Can you work these out from the model? Positions are in its coordinate system, mm. A direction names the side the tool comes from. Coordinates: 2 decimals unless noted, no trailing zeros. Loops run counter-clockwise (first coordinate to the right, second up) from the corner with the lowest first, then second, coordinate; pieces in that order, holes last. Notation, with made-up numbers: M -15.5,-13 L 41.5,-13 A19 ccw 41.5,11 Z; hole C 68,-9 d5. An arc over 180 degrees is marked long. Answer as a JSON object with one key per item and string values. Group by question number.
Item 1: We'd pull the mould along Y, two halves only. Please class faces 1 (the flat face through (0, -2, -22)), 2 (the cylindrical face through (-1.57, -3.86, 5.04)), 3 (the flat face through (-1.565, -54.056, 3.924)): +Y half, -Y half, draft (parallel to the pull), parting line (faces both ways), or undercut.
Item 2: Which directions (+Z, -Z, +X, -X, +Y, -Y) give clear straight access to the entire face, cutting with the end or side of a thin tool? Please do faces 4 (the cylindrical face through (-1.565, -46.994, -15.824)), 5 (the flat face through (-1.565, -44.442, -47.356)).
Item 3: I'm going to push flat-ended pins straight in: pin 1 Ø1 at (x, y) = (-2.5, -20.5) entering from +Z; pin 2 Ø1.5 at (y, z) = (75.5, -40) entering from -X. Where does each tip first touch, or does it pass through?
Item 4: Suppose I cut it at C-C (z = -56.5). Write out the boundary of the cut face in (x, y) (3 decimals).
Item 5: Suppose I cut it at D-D (x = -2.5). Write out the boundary of the cut face in (y, z).
Item 6: If I drill on line 1 (Y direction, x = -0.7, z = -25); line 2 (Y direction, x = -2.7, z = 2.5); line 3 (Y direction, x = -2.15, z = 2), over which ranges is the centre line in solid material (lowest first)?
Item 7: Suppose I cut it at B-B (z = -44). Write out the boundary of the cut face in (x, y) (3 decimals).
Item 8: Suppose I cut it at A-A (y = 0). Write out the boundary of the cut face in (x, z) (3 decimals), then the cut area to 3 significant figures.
```python
from build123d import *

# Parameters (mm, degrees)
SKETCH1_R           = 6.35
SKETCH1_R_2         = 5
BOSS_EXTRUDE1_DEPTH = 3.175


with BuildPart() as part:
    # Sketch1 → Boss-Extrude1 (new body)
    with BuildSketch(Plane.YZ):
        Polygon((-92.963597619, -40.991822572), (-82.715641976, -64.232721977), (-5.080718921, -30), (2.443726878, -30), (78.037119616, -69.842164643), (89.880151319, -47.372126813), (101.723183023, -24.902088983), (7.042880264, 25), (-6.258566793, 25), (-103.211553262, -17.750923167), align=None)
        with Locations(Location((0, 0, 0), (0, 0, 270))):
            Circle(SKETCH1_R, mode=Mode.SUBTRACT)
        with Locations(Location((-81.343147916, -35.867844751, 0), (0, 0, 270))):
            Circle(SKETCH1_R_2, mode=Mode.SUBTRACT)
        with Locations(Location((-47.213795641, -20.818681542, 0), (0, 0, 270))):
            Circle(SKETCH1_R_2, mode=Mode.SUBTRACT)
        with Locations(Location((78.645132405, -41.450610961, 0), (0, 0, 270))):
            Circle(SKETCH1_R_2, mode=Mode.SUBTRACT)
        with Locations(Location((45.647793387, -24.059072279, 0), (0, 0, 270))):
            Circle(SKETCH1_R_2, mode=Mode.SUBTRACT)
    extrude(amount=-BOSS_EXTRUDE1_DEPTH)


solid = part.part
```
From the geometry:
{
 "1": {"face 1": "draft", "face 2": "undercut", "face 3": "-Y half"},
 "2": {"face 4": "+X, -X", "face 5": "-Z, +X, -X"},
 "3": {"pin 1": "z = 18.94", "pin 2": "through"},
 "4": {"outline": "M -3.175,-86.125 L 0,-86.125 L 0,-65.179 L -3.175,-65.179 Z; M -3.175,52.723 L 0,52.723 L 0,85.069 L -3.175,85.069 Z"},
 "5": {"outline": "M -103.21,-17.75 L -82.72,-64.23 L -5.08,-30 L 2.44,-30 L 78.04,-69.84 L 101.72,-24.9 L 7.04,25 L -6.26,25 Z; hole C -81.34,-35.87 d10; hole C -47.21,-20.82 d10; hole C 0,0 d12.7; hole C 45.65,-24.06 d10; hole C 78.65,-41.45 d10"},
 "6": {"line 1": "-100.02 to -49.96, -44.47 to 40.74, 50.56 to 101.67", "line 2": "-57.29 to -5.84, 5.84 to 49.73", "line 3": "-58.42 to -6.03, 6.03 to 50.68"},
 "7": {"outline": "M -3.175,-91.637 L 0,-91.637 L 0,-36.831 L -3.175,-36.831 Z; M -3.175,29.006 L 0,29.006 L 0,74.344 L -3.175,74.344 Z; M -3.175,82.946 L 0,82.946 L 0,91.657 L -3.175,91.657 Z"},
 "8": {"outline": "M -3.175,-30 L 0,-30 L 0,-6.35 L -3.175,-6.35 Z; M -3.175,6.35 L 0,6.35 L 0,25 L -3.175,25 Z", "area": "134 mm2"}
}
